CAD build for the part. Positions are in the model's coordinates, mm. Round coordinates to 2 decimals unless told otherwise and drop trailing zeros. Loops run counter-clockwise (first coordinate to the right, second up) from the corner with the lowest first, then second, coordinate; pieces in that order, holes last. Notation, with made-up numbers: M 2,89.25 L 27,89.25 A10 ccw 27,101.25 Z; hole C -38.75,37.5 d11. An arc over 180 degrees is marked long. Use a Markdown table: item, result. Add a question column.
(1) Flat gauge pin, fed straight in: P1, Ø1.6, axis at x = -218, y = 0.5, coming from the +Z side. Where does the tip first touch, or does it go through?
(2) Band-saw the part on B-B, the plane z = -107. Write the cut outline in (x, y) (1 decimal), and give its area (3 significant figures).
(3) Band-saw the part on A-A, the plane y = 1.1. Write the cut outline in (x, z), and give its area (3 significant figures).
(4) Wall check: L1, parallel to Z at x = 92, y = 0.8; L2, parallel to X at y = -1.4, z = -8; L3, parallel to Z at x = -156.5, y = -0.4. Give the ranges that are in metal, low to high.
(5) Band-saw the part on C-C, the plane x = 203.5. Write the cut outline in (y, z), and give its area (3 significant figures).
from build123d import *

# Parameters (mm, degrees)
BOSS_EXTRUDE1_DEPTH = 1.5875
SKETCH8_R           = 1.4986
SKETCH8_R_2         = 1.489912236
SKETCH8_W           = 55.88
SKETCH8_H           = 20.32
CUT_EXTRUDE1_DEPTH  = 20.32


with BuildPart() as part:
    # Sketch3 → Boss-Extrude1 (new body, symmetric)
    with BuildSketch(Plane(origin=(0, 0, 0), x_dir=(1, 0, 0), z_dir=(0, 1, 0))):
        Polygon((-279.4, 95.25), (-139.7, 95.25), (-120.65, 133.35), (133.35, 133.35), (152.4, 95.25), (279.4, 95.25), (279.4, -95.25), (152.4, -95.25), (133.35, -133.35), (-120.65, -133.35), (-139.7, -95.25), (-279.4, -95.25), align=None)
    extrude(amount=BOSS_EXTRUDE1_DEPTH, both=True)

    # Sketch8 → Cut-Extrude1 (cut)
    with BuildSketch(Plane(origin=(0, 1.5875, 0), x_dir=(1, 0, 0), z_dir=(0, 1, 0))):
        with Locations((136.914734299, 0.595522161)):
            Circle(SKETCH8_R)
        with Locations((41.78446907, -0.595522161)):
            Circle(SKETCH8_R_2)
        with Locations((97.265334299, 0.595522161)):
            Rectangle(SKETCH8_W, SKETCH8_H)
    extrude(amount=-CUT_EXTRUDE1_DEPTH, mode=Mode.SUBTRACT)


solid = part.part
Return value:
| question | item | result |
|---|---|---|
| 1 | P1 | z = 95.25 |
| 2 | outline | M -133.8,-1.6 L 146.5,-1.6 L 146.5,1.6 L -133.8,1.6 Z |
| 2 | area | 890 mm^2 |
| 3 | outline | M -279.4,-95.25 L -139.7,-95.25 L -120.65,-133.35 L 133.35,-133.35 L 152.4,-95.25 L 279.4,-95.25 L 279.4,95.25 L 152.4,95.25 L 133.35,133.35 L -120.65,133.35 L -139.7,95.25 L -279.4,95.25 Z; hole C 41.78,0.6 d2.98; hole M 69.33,-10.76 L 125.21,-10.76 L 125.21,9.56 L 69.33,9.56 Z; hole C 136.91,-0.6 d3 |
| 3 | area | 126,000 mm^2 |
| 4 | L1 | -133.35 to -10.76, 9.56 to 133.35 |
| 4 | L2 | -279.4 to 69.33, 125.21 to 279.4 |
| 4 | L3 | -95.25 to 95.25 |
| 5 | outline | M -1.59,-95.25 L 1.59,-95.25 L 1.59,95.25 L -1.59,95.25 Z |
| 5 | area | 605 mm^2 |
